The drawing under review shows one solid part. Ordinate dimensions are in mm from its lowest x, y, z. A direction names the side the tool comes from. Round coordinates to 2 decimals unless told otherwise and drop trailing zeros. Order: outer loops, then holes, each group sorted by start corner. A loop starts at its lowest first (then second) coordinate and runs counter-clockwise, first axis right, second up. Notation, with made-up numbers: M -11,38.25 L 11,38.25 A19 ccw 11,65.25 Z; hole C 49,51.5 d10. An arc over 180 degrees is marked long. Use a Markdown table: item, result.
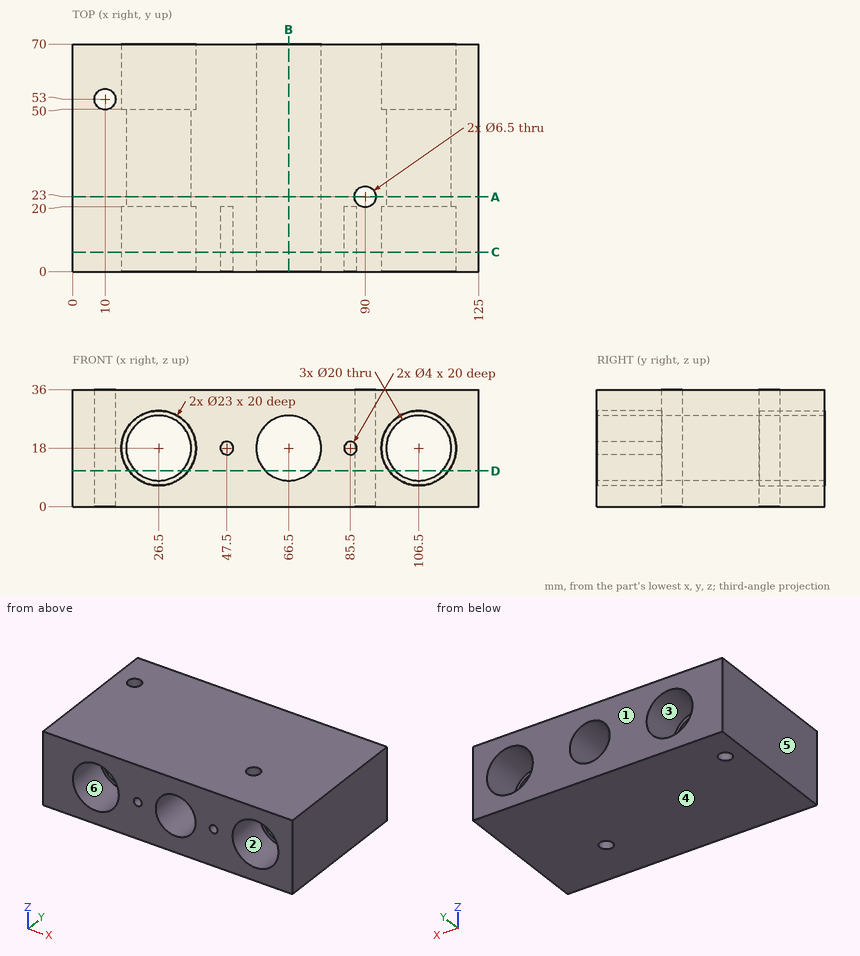
Q1. Add section A-A (y = 23). Write out the cut boundary in (x, z).
Determined:
| item | result |
|---|---|
| outline | M 0,0 L 86.75,0 L 86.75,36 L 0,36 Z; M 93.25,0 L 125,0 L 125,36 L 93.25,36 Z; hole C 26.5,18 d20; hole C 66.5,18 d20; hole C 106.5,18 d20 |
Q2. Draft analysis for pull direction Z (two halves, no side actions). For the marked faces 4, 5 and 6, state which applies: pulls with the +Z half, pulls with the -Z half, needs draft (parallel to the pull), parting line crosses it, or undercut.
Determined:
| item | result |
|---|---|
| face 4 | pulls with the -Z half |
| face 5 | needs draft |
| face 6 | undercut |
Q3. Clearance check with flat-ended pins moving along their axes: pin 1 (20.5 mm diameter, centred on x = 106.5, z = 18, fed in from +Y); pin 2 (1.5 mm diameter, centred on x = 79, z = 23.5, fed in from -Y); pin 3 (10 mm diameter, centred on x = 21.5, z = 19, fed in from -Y); pin 4 (7 mm diameter, centred on x = 102.5, z = 14.5, fed in from +Y). State where each tip first meets the part, or that it passes through.
Determined:
| item | result |
|---|---|
| pin 1 | stops at y = 50 |
| pin 2 | stops at y = 0 |
| pin 3 | stops at y = 20 |
| pin 4 | passes through |
Q4. Machinability: for the marked faces 1, 2 and 3, which of the approach directions +Z, -Z, +X, -X, +Y, -Y give a long, thin tool a straight path to every point of the face, cutting with its end or side? Answer none if there is none.
Determined:
| item | result |
|---|---|
| face 1 | +Z, -Z, +X, -X, +Y |
| face 2 | -Y |
| face 3 | +Y |
Q5. Add section B-B (x = 66.5). Write out the cut boundary in (y, z), then the cut area to 3 significant figures.
Determined:
| item | result |
|---|---|
| outline | M 0,0 L 70,0 L 70,8 L 0,8 Z; M 0,28 L 70,28 L 70,36 L 0,36 Z |
| area | 1,120 mm^2 |
Q6. Add section D-D (z = 11). Give the number of separate pieces and of enclosed holes in the cut face, then the cut area to 3 significant figures.
Determined:
| item | result |
|---|---|
| separate pieces | 4 |
| enclosed holes | 2 |
| area | 5,370 mm^2 |
Q7. Add section C-C (y = 6). Write out the cut boundary in (x, z), then the cut area to 3 significant figures.
Determined:
| item | result |
|---|---|
| outline | M 0,0 L 125,0 L 125,36 L 0,36 Z; hole C 26.5,18 d23; hole C 47.5,18 d4; hole C 66.5,18 d20; hole C 85.5,18 d4; hole C 106.5,18 d23 |
| area | 3,330 mm^2 |
Q8. Wall thickness on line 1 along X through (y, z) = (25, 17.5); line 2 along Y through (x, z) = (90, 28); line 3 along X through (y, z) = (59.5, 20): over which ranges is each line inside the solid? List them lowest first. Write a range as [from, to].
Determined:
| item | result |
|---|---|
| line 1 | x = [0, 16.51], [36.49, 56.51], [76.49, 87.44], [92.56, 96.51], [116.49, 125] |
| line 2 | y = [0, 19.75], [26.25, 70] |
| line 3 | x = [0, 15.18], [37.82, 56.7], [76.3, 95.18], [117.82, 125] |
